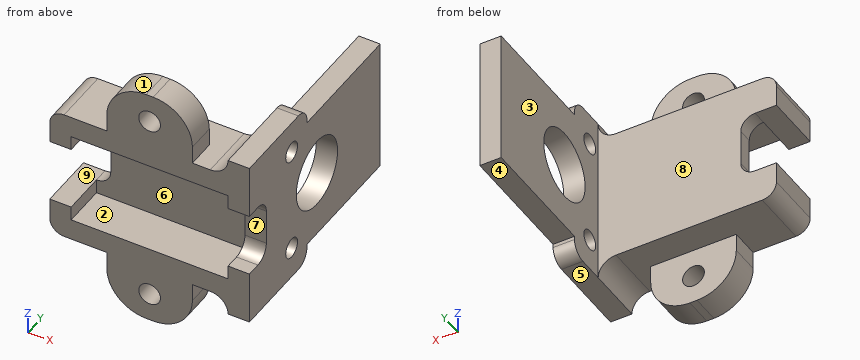
```python
from build123d import *

# Parameters (mm, degrees)
SKETCH1_W           = 22
SKETCH1_H           = 13
BOSS_EXTRUDE1_DEPTH = 6
BOSS_EXTRUDE2_DEPTH = 2
BOSS_EXTRUDE3_DEPTH = 8
SKETCH4_R           = 1.525
SKETCH4_R_2         = 1.524
CUT_EXTRUDE1_DEPTH  = 36.566838488
SKETCH5_W           = 9
SKETCH5_H           = 4
CUT_EXTRUDE2_DEPTH  = 38.735924528
FILLET1_R           = 2
SKETCH6_W           = 12
SKETCH6_H           = 13.009000019
SKETCH6_W_2         = 15.838286437
CUT_EXTRUDE3_DEPTH  = 4
BOSS_EXTRUDE4_DEPTH = 23
CUT_EXTRUDE4_DEPTH  = 23
SKETCH9_R           = 4.9
CUT_EXTRUDE6_DEPTH  = 23
SKETCH10_R          = 1.4
CUT_EXTRUDE7_DEPTH  = 23
BOSS_EXTRUDE5_DEPTH = 3
FILLET2_R           = 2.5
FILLET3_R           = 2.5


with BuildPart() as part:
    # Sketch1 → Boss-Extrude1 (new body)
    with BuildSketch(Plane(origin=(0, 0, 0), x_dir=(1, 0, 0), z_dir=(0, 1, 0))):
        with BuildLine():
            Line((-1, -3), (23, -3))
            Line((23, -3), (25, -3))
            Line((25, -3), (25, -1))
            Line((25, -1), (25, 14))
            Line((25, 14), (25, 16))
            Line((25, 16), (23, 16))
            Line((23, 16), (-1, 16))
            ThreePointArc((-1, 16), (-2.414213562, 15.414213562), (-3, 14))
            Line((-3, 14), (-3, -1))
            ThreePointArc((-3, -1), (-2.414213562, -2.414213562), (-1, -3))
        make_face()
        with Locations((11, 6.5)):
            Rectangle(SKETCH1_W, SKETCH1_H, mode=Mode.SUBTRACT)
    extrude(amount=BOSS_EXTRUDE1_DEPTH)

    # Sketch2 → Boss-Extrude2 (add)
    with BuildSketch(Plane(origin=(0, 6, 0), x_dir=(1, 0, 0), z_dir=(0, 1, 0))):
        with BuildLine():
            Line((25, 14), (25, -1))
            Line((25, -1), (25, -3))
            Line((25, -3), (23, -3))
            Line((23, -3), (-1, -3))
            ThreePointArc((-1, -3), (-2.414213562, -2.414213562), (-3, -1))
            Line((-3, -1), (-3, 14))
            ThreePointArc((-3, 14), (-2.414213562, 15.414213562), (-1, 16))
            Line((-1, 16), (23, 16))
            Line((23, 16), (25, 16))
            Line((25, 16), (25, 14))
        make_face()
    extrude(amount=BOSS_EXTRUDE2_DEPTH)

    # Sketch3 → Boss-Extrude3 (add)
    with BuildSketch(Plane.XZ):
        with BuildLine():
            Line((5, 3), (17, 3))
            Line((17, 3), (17, 5.5))
            ThreePointArc((17, 5.5), (15.389087297, 9.389087297), (11.5, 11))
            Line((11.5, 11), (10.5, 11))
            ThreePointArc((10.5, 11), (6.610912703, 9.389087297), (5, 5.5))
            Line((5, 5.5), (5, 3))
        make_face()
        with BuildLine():
            Line((17, -16), (5, -16))
            Line((5, -16), (5, -18.5))
            ThreePointArc((5, -18.5), (6.610912703, -22.389087297), (10.5, -24))
            Line((10.5, -24), (11.5, -24))
            ThreePointArc((11.5, -24), (15.389087297, -22.389087297), (17, -18.5))
            Line((17, -18.5), (17, -16))
        make_face()
    extrude(amount=-BOSS_EXTRUDE3_DEPTH)

    # Sketch4 → Cut-Extrude1 (cut, through all)
    with BuildSketch(Plane(origin=(0, 0, 0), x_dir=(-1, 0, 0), z_dir=(0, -1, 0))):
        with Locations(Location((-11, 20, 0), (0, 0, 90))):
            Circle(SKETCH4_R)
        with Locations(Location((-11, -7, 0), (0, 0, 90))):
            Circle(SKETCH4_R_2)
    extrude(amount=-CUT_EXTRUDE1_DEPTH, mode=Mode.SUBTRACT)

    # Sketch5 → Cut-Extrude2 (cut, through all)
    with BuildSketch(Plane(origin=(25, 0, 0), x_dir=(0, 0, -1), z_dir=(1, 0, 0))):
        with Locations((6.5, 2)):
            Rectangle(SKETCH5_W, SKETCH5_H)
    extrude(amount=-CUT_EXTRUDE2_DEPTH, mode=Mode.SUBTRACT)

    # Fillet1
    fillet1_edges = [part.edges().sort_by_distance(p)[0] for p in [
        (-1.5, 4, -11),
        (-1.5, 4, -2),
        (23.5, 4, -11),
        (23.5, 4, -2),
    ]]
    fillet(fillet1_edges, radius=FILLET1_R)

    # Sketch6 → Cut-Extrude3 (cut)
    with BuildSketch(Plane(origin=(0, 8, 0), x_dir=(1, 0, 0), z_dir=(0, 1, 0))):
        with Locations((11, 22.504500009)):
            Rectangle(SKETCH6_W, SKETCH6_H)
        with Locations((11.149066226, -9.50450001)):
            Rectangle(SKETCH6_W_2, SKETCH6_H)
    extrude(amount=-CUT_EXTRUDE3_DEPTH, mode=Mode.SUBTRACT)

    # Sketch7 → Boss-Extrude4 (add)
    with BuildSketch(Plane(origin=(0, 8, 0), x_dir=(1, 0, 0), z_dir=(0, 1, 0))):
        Polygon((23, 16), (22, 16), (22, -3), (23, -3), (25, -3), (25, -1), (25, 14), (25, 16), align=None)
    extrude(amount=BOSS_EXTRUDE4_DEPTH)

    # Sketch8 → Cut-Extrude4 (cut)
    with BuildSketch(Plane(origin=(0, 8, 0), x_dir=(1, 0, 0), z_dir=(0, 1, 0))):
        with BuildLine():
            Line((-3, 2), (0, 2))
            ThreePointArc((0, 2), (1.414213562, 2.585786438), (2, 4))
            Line((2, 4), (2, 9))
            ThreePointArc((2, 9), (1.414213562, 10.414213562), (0, 11))
            Line((0, 11), (-3, 11))
            Line((-3, 11), (-3, 2))
        make_face()
    extrude(amount=-CUT_EXTRUDE4_DEPTH, mode=Mode.SUBTRACT)

    # Sketch9 → Cut-Extrude6 (cut)
    with BuildSketch(Plane.ZY.offset(-22)):
        with Locations((-6.5, 16)):
            Circle(SKETCH9_R)
    extrude(amount=-CUT_EXTRUDE6_DEPTH, mode=Mode.SUBTRACT)

    # Sketch10 → Cut-Extrude7 (cut)
    with BuildSketch(Plane.ZY.offset(-22)):
        with Locations((-14, 10)):
            Circle(SKETCH10_R)
        with Locations((1, 10)):
            Circle(SKETCH10_R)
    extrude(amount=-CUT_EXTRUDE7_DEPTH, mode=Mode.SUBTRACT)

    # Sketch11 → Boss-Extrude5 (add)
    with BuildSketch(Plane(origin=(25, 0, 0), x_dir=(0, 0, -1), z_dir=(1, 0, 0))):
        with BuildLine():
            Line((-3, 0), (-5.5, 0))
            Line((-5.5, 0), (-5.5, 11.617902622))
            ThreePointArc((-5.5, 11.617902622), (-4.914213562, 13.032116185), (-3.5, 13.617902622))
            Line((-3.5, 13.617902622), (-3, 13.617902622))
            Line((-3, 13.617902622), (-3, 0))
        make_face()
        with BuildLine():
            Line((16, 0), (18.5, 0))
            Line((18.5, 0), (18.5, 11.617902622))
            ThreePointArc((18.5, 11.617902622), (17.914213562, 13.032116185), (16.5, 13.617902622))
            Line((16.5, 13.617902622), (16, 13.617902622))
            Line((16, 13.617902622), (16, 0))
        make_face()
    extrude(amount=-BOSS_EXTRUDE5_DEPTH)

    # Fillet2
    fillet2_edges = [part.edges().sort_by_distance(p)[0] for p in [
        (22, 4, 3),
    ]]
    fillet(fillet2_edges, radius=FILLET2_R - 0.0001)  # a hair under: the kernel refuses the full size

    # Fillet3
    fillet3_edges = [part.edges().sort_by_distance(p)[0] for p in [
        (22, 4, -16),
    ]]
    fillet(fillet3_edges, radius=FILLET3_R - 0.0001)  # a hair under: the kernel refuses the full size


solid = part.part
```
Input: part model. Units: mm. Frame: model coordinates. Face numbers are marked on the shaded views. A direction names the side the tool comes from. Give positions to 0.01 mm unless a question says otherwise; leave off trailing zeros. Order: outer loops, then holes, each group sorted by start corner. A loop starts at its lowest first (then second) coordinate and runs counter-clockwise, first axis right, second up.
1. Cut plane A-A (y = 10). Return loops of the section in (x, z), and give its area (3 significant figures).
Computed:
outline: (22, -18.5) - (25, -18.5) - (25, -15.4) - (22, -15.4) - close; (22, -12.6) - (25, -12.6) - (25, -0.4) - (22, -0.4) - close; (22, 2.4) - (25, 2.4) - (25, 5.5) - (22, 5.5) - close
area: 55.2 mm2
2. Set-up query: the marked faces 5, 6, 7, 8 and 9. Return all of +Z, -Z, +X, -X, +Y, -Y with unobstructed straight access to the full face (end or side cutting, diameter ignored); none if empty.
Computed:
face 5: -Z, +X, +Y, -Y
face 6: -Y
face 7: +X, -X, -Y
face 8: +Z, -Z, -X, +Y
face 9: -X, +Y, -Y
3. Pin query (flat end, axial travel): pin 1 Ø6 at (y, z) = (5.5, -18.5) entering from -X; pin 2 Ø3.5 at (x, y) = (23, 20) entering from -Z; pin 3 Ø3 at (x, y) = (19.5, 19) entering from +Z; pin 4 Ø1 at (y, z) = (7.5, -7.5) entering from -X. Return the tip coordinate at first contact, or that it passes through.
Computed:
pin 1: stops at x = -2.32
pin 2: stops at z = -16
pin 3: passes through
pin 4: stops at x = 2
4. Line query: probe 1 along Y at (x, z) = (23.9, -14); probe 2 along Y at (x, z) = (-1.25, -11.5); probe 3 along Y at (x, z) = (13, 4). Output: solid intervals per line, ascending.
Computed:
probe 1: y = 0 to 8.6, 11.4 to 31
probe 2: y = 0 to 8
probe 3: y = 0 to 4
5. Draft query along Z for the marked faces 1, 2, 3 and 4. Return one class per face: released by +Z, released by -Z, zero draft, split by the parting line, or undercut.
Computed:
face 1: released by +Z
face 2: undercut
face 3: zero draft
face 4: released by -Z
6. Cut plane B-B (z = -6.5). Return loops of the section in (x, y).
Computed:
outline: (2, 6) - (22, 6) - (22, 4) - (25, 4) - (25, 11.1) - (22, 11.1) - (22, 8) - (2, 8) - close; (22, 20.9) - (25, 20.9) - (25, 31) - (22, 31) - close
7. Cut plane D-D (x = 1). Return loops of the section in (y, z), and give its area (3 significant figures).
Computed:
outline: (0, -16) - (8, -16) - (8, -10.73) - (6, -10.73) - (6, -13) - (0, -13) - close; (0, 0) - (6, 0) - (6, -2.27) - (8, -2.27) - (8, 3) - (0, 3) - close
area: 57.1 mm2
8. Cut plane C-C (z = -12). Return loops of the section in (x, y), and give its area (3 significant figures).
Computed:
outline: (-3, 0) - (0, 0) - (0, 6) - (22, 6) - (22, 0) - (25, 0) - (25, 31) - (22, 31) - (22, 8) - (-3, 8) - close
area: 161 mm2
